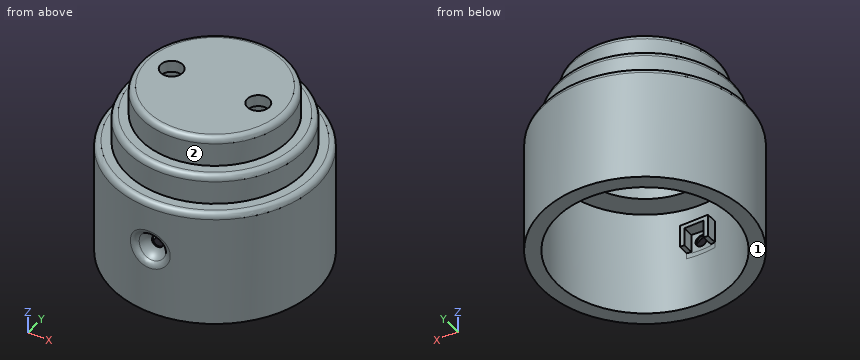
Autodesk Inventor part; units mm, degrees
ref_plane "Work Plane2" through (0, 0, 35) normal (0, 0, 1) x (1, 0, 0)
ref_plane "Work Plane3" through (0, 0, 40) normal (0, 0, 1) x (1, 0, 0)
ref_plane "Work Plane4" through (0, 0, 60) normal (0, 0, 1) x (1, 0, 0)
sketch "Sketch1" plane through (0, 0, 0) normal (0, 0, 1) x (1, 0, 0)
  point P0 (0, 0)
sketch "Sketch2" plane through (0, 0, 0) normal (0, 0, 1) x (1, 0, 0)
  circle A0 centre (0, 0) radius 35
  dimension "d0" = 70
ref_plane "Work Plane1" through (0, 0, 30) normal (0, 0, 1) x (1, 0, 0)
sketch "Sketch3" plane through (0, 0, 30) normal (0, 0, 1) x (1, 0, 0)
  circle A0 centre (0, 0) radius 30
  dimension "d3" = 60
ref_plane "Work Plane2" through (0, 0, 35) normal (0, 0, 1) x (1, 0, 0)
sketch "Sketch4" plane through (0, 0, 35) normal (0, 0, 1) x (1, 0, 0)
  circle A0 centre (0, 0) radius 25
  dimension "d7" = 50
extrude "Extrusion1" add sketch "Sketch2" along normal blind 40
fillet "Fillet2" radius 2 1 edges at (-35, 0, 40)
ref_plane "Work Plane3" through (0, 0, 40) normal (0, 0, 1) x (1, 0, 0)
sketch "Sketch9" plane through (0, 0, 40) normal (0, 0, 1) x (1, 0, 0)
  circle A0 centre (0, 0) radius 33
  circle A1 centre (0, 0) radius 30
  dimension "d42" = 60
extrude "Extrusion8" add sketch "Sketch9" along normal blind 10 contours A1
sketch "Sketch10" plane through (0, 0, 50) normal (0, 0, 1) x (1, 0, 0)
  circle A0 centre (0, 0) radius 30
  circle A1 centre (0, 0) radius 25
  dimension "d45" = 50
extrude "Extrusion9" add sketch "Sketch10" along normal blind 10 contours A1
sketch "Sketch11" plane through (0, 0, 60) normal (0, 0, 1) x (1, 0, 0)
  circle A0 centre (0, 0) radius 25
  circle A1 centre (0, 0) radius 22.5
  dimension "d48" = 45
extrude "Extrusion10" cut sketch "Sketch11" against normal blind 60 contours A1
sketch "Sketch14" plane through (0, 0, 0) normal (0, 0, -1) x (-1, 0, 0)
  circle A0 centre (0, 0) radius 22.5
  circle A1 centre (0, 0) radius 35
  circle A2 centre (0, 0) radius 30
  dimension "d58" = 60
extrude "Extrusion12" cut sketch "Sketch14" against normal blind 36 contours A2
sketch "Sketch15" plane through (0, 0, 36) normal (0, 0, -1) x (-1, 0, 0)
  circle A0 centre (0, 0) radius 22.5
  circle A1 centre (0, 0) radius 30
ref_plane "Work Plane4" through (0, 0, 60) normal (0, 0, 1) x (1, 0, 0)
sketch "Sketch18" plane through (0, 0, 60) normal (0, 0, 1) x (1, 0, 0)
  circle A0 centre (-14.95, 0) radius 3.75
  line L0 (-49, 0) -> (49, 0)
  line L1 (0, -49) -> (0, 49)
  circle A1 centre (14.95, 0) radius 3.75
  circle A2 centre (0, 0) radius 22.5
  point P0 (22.5, 0)
  point P1 (-11.2, 0)
  point P2 (10.775, 0)
  dimension "d71" = 7.5
  dimension "d78" = 14.95
  dimension "d81" = 45
extrude "Extrusion16" add sketch "Sketch18" against normal blind 4 contours L0 L1 A2 A0 | A0 L0 A2 L1 | L1 A2 L0 A1 | L0 A1 A2 L1
fillet "Fillet5" radius 2 2 edges at (-30, 0, 50) (-25, 0, 60)
ref_plane "Work Plane5" through (0, -35, 0) normal (0, 1, 0) x (-1, 0, 0)
sketch "Sketch19" plane through (0, -35, 0) normal (0, 1, 0) x (-1, 0, 0)
  line L0 (49, 0) -> (-49, 0)
  line L1 (0, -12) -> (0, 72)
  arc A0 (0, 27.857143) -> (0, 17.857143) centre (0, 22.857143) ccw
  line L2 (0, 27.857143) -> (0, 17.857143)
  point P0 (0, 0)
  dimension "d86" = 10
revolve "Revolution1" cut sketch "Sketch19" angle 360 about axis through (0, -35, -10) along (0, 0, 1)
ref_plane "Work Plane6" through (0, -35, 0) normal (0, 1, 0) x (-1, 0, 0)
sketch "Sketch20" plane through (0, -35, 0) normal (0, 1, 0) x (-1, 0, 0)
  line L0 (0, -12) -> (0, 72)
  line L1 (49, 0) -> (-49, 0)
  line L2 (0, 27.857143) -> (0, 17.857143)
  circle A0 centre (0, 22.857143) radius 2
  point P0 (0, 0)
  dimension "d90" = 4
extrude "Extrusion17" cut sketch "Sketch20" along normal blind 10
ref_plane "Work Plane7" through (0, -29, 0) normal (0, 1, 0) x (-1, 0, 0)
sketch "Sketch21" plane through (0, -29, 0) normal (0, 1, 0) x (-1, 0, 0)
  line L0 (-4.85, 27.7) -> (4.85, 27.7)
  line L1 (4.85, 27.7) -> (4.85, 18)
  line L2 (4.85, 18) -> (-4.85, 18)
  line L3 (-4.85, 18) -> (-4.85, 27.7)
  line L4 (-3.35, 26.2) -> (3.35, 26.2)
  line L5 (3.35, 26.2) -> (3.35, 19.5)
  line L6 (3.35, 19.5) -> (-3.35, 19.5)
  line L7 (-3.35, 19.5) -> (-3.35, 26.2)
  line L8 (-35, 0) -> (35, 0)
  line L9 (-49, 0) -> (49, 0)
  line L10 (49, 0) -> (-49, 0)
  line L11 (0, -12) -> (0, 72)
  point P0 (0, 0)
  dimension "d99" = 18
  dimension "d101" = 6.7
  dimension "d102" = 1.5
  dimension "d103" = 1.5
  dimension "d104" = 1.5
  dimension "d105" = 6.7
extrude "Extrusion18" add sketch "Sketch21" along normal blind 3 and the other way blind 2 contours L0 L11 L4 L7 L6 L2 L3 | L0 L1 L2 L11 L6 L5 L4
fillet "Fillet6" radius 2 2 edges at (-4.9872, -34.6429, 22.8521) (4.9872, -34.6429, 22.8557)
sketch "Sketch22" plane through (0, 0, 18) normal (0, 0, -1) x (-1, 0, 0)
  arc A0 (-4.85, -29.605363) -> (4.85, -29.605363) centre (0, 0) ccw
  line L0 (-4.85, -26) -> (-4.85, -29.605363)
  line L1 (-4.85, -26) -> (4.85, -26)
  line L2 (4.85, -26) -> (4.85, -29.605363)
  line L3 (-4.85, -29.605363) -> (-4.85, -26)
  arc A1 (-4.85, -29.605363) -> (4.85, -29.605363) centre (0, -1.266986) ccw
sketch "Sketch22 outline for Extrusion19" plane through (0, 0, 18) normal (0, 0, -1) x (-1, 0, 0)
  line L0 (-4.85, -26) -> (-4.85, -29.605363)
  line L1 (4.85, -26) -> (-4.85, -26)
  line L2 (4.85, -29.605363) -> (4.85, -26)
  arc A0 (-4.85, -29.605363) -> (4.85, -29.605363) centre (0, 0) ccw
extrude "Extrusion19" cut sketch "Sketch22 outline for Extrusion19" against normal blind 2
sketch "Sketch23" plane through (0, -26, 0) normal (0, 1, 0) x (1, 0, 0)
  line L0 (4.85, -20) -> (3.35, -20)
  line L1 (3.35, -20) -> (3.35, -26.2)
  line L2 (3.35, -26.2) -> (-3.35, -26.2)
  line L3 (-3.35, -26.2) -> (-3.35, -20)
  line L4 (-3.35, -20) -> (-4.85, -20)
  line L5 (-4.85, -20) -> (-4.85, -27.7)
  line L6 (-4.85, -27.7) -> (4.85, -27.7)
  line L7 (4.85, -27.7) -> (4.85, -20)
  line L8 (-3.35, -21.72852) -> (3.35, -21.72852)
  line L9 (3.35, -21.72852) -> (3.35, -26.2)
  line L10 (3.35, -26.2) -> (-3.35, -26.2)
  line L11 (-3.35, -26.2) -> (-3.35, -21.72852)
  point P0 (0, 0)
properties part number "Carcasa"
Input: part model. Units: mm. Frame: model coordinates. Face numbers are marked on the shaded views. A direction names the side the tool comes from. Round coordinates to 2 decimals unless told otherwise and drop trailing zeros. Write each loop counter-clockwise with the first axis right and the second up, starting at its lowest first coordinate (ties: lowest second). Pieces come first, ordered by that corner, then holes.
1) Ray query, L1, parallel to Z at x = 0, y = -30.2; L2, parallel to Z at x = 3, y = 15; L3, parallel to Z at x = 10.5, y = -31. Return the intervals inside material, ascending.
2) Cut plane A-A (y = 0). Count the separate pieces of the cut face and the enclosed holes in it, then the cut area to 3 significant figures.
3) Cut plane B-B (z = 39). Return the cut outline in (x, y).
4) Reachability of the marked faces 1 and 2 from +Z, -Z, +X, -X, +Y, -Y: full face, straight path, thin tool, end or side. Return the list, or none.
5) Contact query for flat-ended pins moving along their axis: P1, Ø13.5, axis at x = 8.5, y = -3.5, coming from the -Z side; P2, Ø2, axis at x = 12, z = 23, coming from the -Y side; P3, Ø1.1, axis at y = -28, z = 21.5, coming from the -X side; P4, Ø7, axis at x = -14.95, y = 0, coming from the +Z side. Output: stop coordinate, or through.
Geometry says:
1. L1: z = 0 to 20.86, 24.86 to 40
1. L2: z = 56 to 60
1. L3: z = 0 to 40
2. separate pieces: 3
2. enclosed holes: 0
2. area: 775 mm2
3. outline: circle Ø69.46 at (0, 0); hole circle Ø45 at (0, 0)
4. face 1: -Z, +X, -X, +Y, -Y
4. face 2: +Z
5. P1: stops at z = 56
5. P2: stops at y = -33.23
5. P3: stops at x = -21.71
5. P4: passes through
